The listing builds one solid part. Answer for the finished solid, in the listing's coordinates (mm). A direction names the side the tool comes from. Round coordinates to 2 decimals unless told otherwise and drop trailing zeros. Write each loop counter-clockwise with the first axis right and the second up, starting at its lowest first coordinate (ties: lowest second). Pieces come first, ordered by that corner, then holes. Notation, with made-up numbers: (-16, -25.75) - (7, -25.75) arc R26 cw to (7, -8.75) - close; hole circle Ø5 at (88.25, 69.25). An arc over 180 degrees is marked (long way). Answer as CSV lines item,"result". Start each with the question number.
Item 1: A cutting plane is placed at C-C on z = -9. Determine the outline of the cut face in (x, y).
Item 2: Straight lines are drawn through the part: line 1 along X through (y, z) = (29, 2.5); line 2 along Y through (x, z) = (8.5, 3.75); line 3 along Y through (x, z) = (3, -10.25). For each, find the intervals that lie inside material, in ascending order. Write a range as [from, to].
Item 3: Flat-ended cylindrical pins translate along their axes: pin 1 (6 mm diameter, centred on x = 0, y = 30, fed in from -Z); pin 2 (4 mm diameter, centred on x = -6, z = -11.5, fed in from +Y); pin 3 (6 mm diameter, centred on y = 33, z = 8, fed in from +X); pin 4 (8 mm diameter, centred on y = 16.5, z = -4, fed in from -X). Find the tip coordinate at first contact, or state that the pin passes through.
Item 4: For a pull along Y with two mould halves and no side action, classify faces 1 (the flat face through (0, 0, 0)), 2 (the flat face through (14, 16, 0)), 3 (the cylindrical face through (0, 40, 0)), 4 (the flat face through (-20, 5, 0)) as pulls with the +Y half, pulls with the -Y half, needs draft (parallel to the pull), parting line crosses it, or undercut.
Item 5: Which of the six approach directions +Z, -Z, +X, -X, +Y, -Y give full straight-line access (tool end or side, diameter ignored) to faces 5 (the flat face through (-13, 17, 0)), 6 (the flat face through (0, 16, -15))?
Item 6: A cutting plane is placed at A-A on x = 0. Determine the outline of the cut face in (y, z), and give its area (3 significant figures).
Item 7: A cutting plane is placed at D-D on x = -16. Determine the outline of the cut face in (y, z), and give its area (3 significant figures).
Item 8: A cutting plane is placed at B-B on y = 30. Determine the outline of the cut face in (x, z).
```python
from build123d import *

# Parameters (mm, degrees)
ESBO_O1_R                = 5
RESSALTO_EXTRUS_O1_DEPTH = 15


with BuildPart() as part:
    # Esboço1 → Ressalto-extrusão1 (new body, symmetric)
    with BuildSketch(Plane.XY):
        with BuildLine():
            Line((-20, 0), (20, 0))
            Line((20, 0), (20, 10))
            Line((20, 10), (7.071067812, 22.928932188))
            ThreePointArc((7.071067812, 22.928932188), (0, 40), (-7.071067812, 22.928932188))
            Line((-7.071067812, 22.928932188), (-20, 10))
            Line((-20, 10), (-20, 0))
        make_face()
        with Locations((0, 30)):
            Circle(ESBO_O1_R, mode=Mode.SUBTRACT)
    extrude(amount=RESSALTO_EXTRUS_O1_DEPTH, both=True)


solid = part.part
```
Geometry says:
1,outline,"(-20, 0) - (20, 0) - (20, 10) - (7.07, 22.93) arc R10 ccw (long way) to (-7.07, 22.93) - (-20, 10) - close; hole circle Ø10 at (0, 30)"
2,line 1,"x = [-9.95, -4.9], [4.9, 9.95]"
2,line 2,"y = [0, 21.5], [24.73, 35.27]"
2,line 3,"y = [0, 26], [34, 39.54]"
3,pin 1,"passes through"
3,pin 2,"stops at y = 39.17"
3,pin 3,"stops at x = 10"
3,pin 4,"stops at x = -17.5"
4,face 1,"pulls with the -Y half"
4,face 2,"undercut"
4,face 3,"undercut"
4,face 4,"needs draft"
5,face 5,"+Z, -Z, -X"
5,face 6,"-Z, +X, -X, +Y, -Y"
6,outline,"(0, -15) - (25, -15) - (25, 15) - (0, 15) - close; (35, -15) - (40, -15) - (40, 15) - (35, 15) - close"
6,area,"900 mm^2"
7,outline,"(0, -15) - (14, -15) - (14, 15) - (0, 15) - close"
7,area,"420 mm^2"
8,outline,"(-10, -15) - (-5, -15) - (-5, 15) - (-10, 15) - close; (5, -15) - (10, -15) - (10, 15) - (5, 15) - close"
